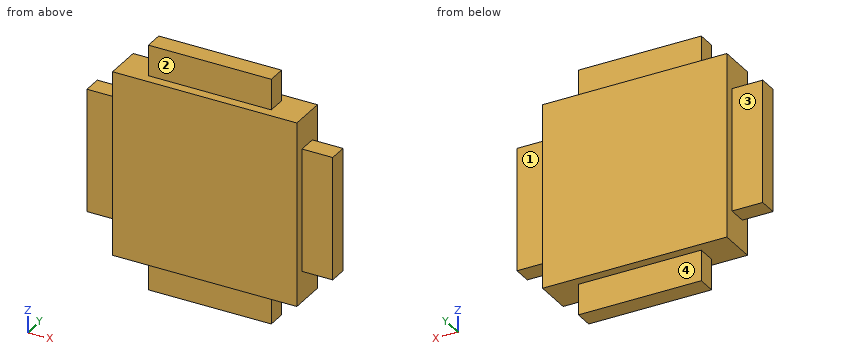
from build123d import *

# Parameters (mm, degrees)
SKETCH1_W                = 15
SKETCH1_H                = 15
BOSS_EXTRUDE2_DEPTH      = 3
SKETCH4_W                = 2.5
SKETCH4_H                = 10
SKETCH4_W_2              = 10
SKETCH4_H_2              = 2.5
BOSS_EXTRUDE3_DEPTH      = 0.75
BOSS_EXTRUDE3_DEPTH_BACK = 0.75


with BuildPart() as part:
    # Sketch1 → Boss-Extrude2 (new body)
    with BuildSketch(Plane(origin=(0, 0, 0), x_dir=(1, 0, 0), z_dir=(0, 1, 0))):
        Rectangle(SKETCH1_W, SKETCH1_H)
    extrude(amount=BOSS_EXTRUDE2_DEPTH)

    # Sketch4 → Boss-Extrude3 (add, two sides)
    with BuildSketch(Plane(origin=(0, 1.5, 0), x_dir=(1, 0, 0), z_dir=(0, 1, 0))) as boss_extrude3_sk:
        with Locations((-8.75, 0)):
            Rectangle(SKETCH4_W, SKETCH4_H)
        with Locations((0, -8.75)):
            Rectangle(SKETCH4_W_2, SKETCH4_H_2)
        with Locations((8.75, 0)):
            Rectangle(SKETCH4_W, SKETCH4_H)
        with Locations((0, 8.75)):
            Rectangle(SKETCH4_W_2, SKETCH4_H_2)
    extrude(amount=BOSS_EXTRUDE3_DEPTH)
    extrude(boss_extrude3_sk.sketch, amount=-BOSS_EXTRUDE3_DEPTH_BACK)


solid = part.part
Geometry: final body of the model. Coordinates: model frame, mm. Face numbers are marked on the shaded views. A direction names the side the tool comes from. Give positions to 0.01 mm unless a question says otherwise; leave off trailing zeros. Loops run counter-clockwise (first coordinate to the right, second up) from the corner with the lowest first, then second, coordinate; pieces in that order, holes last. Notation, with made-up numbers: (-16, 83.25) - (19, 83.25) arc R24 cw to (19, 122.25) - close; hole circle Ø10 at (-27, 36.5). An arc over 180 degrees is marked (long way). Answer as CSV lines item,"result". Start each with the question number.
1. Section B-B, the plane z = -1.75. Return loops of the section in (x, y), plus the area to 3 significant figures.
2. Pin query (flat end, axial travel): P1, Ø2, axis at x = -1.5, z = -9, coming from the -Y side; P2, Ø3, axis at x = -7, z = -1, coming from the -Y side; P3, Ø1.6, axis at y = 1.5, z = 8.5, coming from the -X side; P4, Ø1.2, axis at y = 1, z = -9.5, coming from the +X side. Return the tip coordinate at first contact, or that it passes through.
3. Ray query, L1, parallel to Z at x = -9, y = 2.15; L2, parallel to Z at x = -5, y = 2.3. Return the intervals inside material, ascending.
4. Section C-C, the plane y = 1.4. Return loops of the section in (x, z).
5. Reachability of the marked faces 1, 2, 3 and 4 from +Z, -Z, +X, -X, +Y, -Y: full face, straight path, thin tool, end or side. Return the list, or none.
6. Section A-A, the plane x = 2.25. Return loops of the section in (y, z), plus the area to 3 significant figures.
7. Section D-D, the plane z = 8.25. Return loops of the section in (x, y).
Answers:
1,outline,"(-10, 0.75) - (-7.5, 0.75) - (-7.5, 0) - (7.5, 0) - (7.5, 0.75) - (10, 0.75) - (10, 2.25) - (7.5, 2.25) - (7.5, 3) - (-7.5, 3) - (-7.5, 2.25) - (-10, 2.25) - close"
1,area,"52.5 mm2"
2,P1,"stops at y = 0.75"
2,P2,"stops at y = 0"
2,P3,"stops at x = -5"
2,P4,"stops at x = 5"
3,L1,"z = -5 to 5"
3,L2,"z = -7.5 to 7.5"
4,outline,"(-10, -5) - (-7.5, -5) - (-7.5, -7.5) - (-5, -7.5) - (-5, -10) - (5, -10) - (5, -7.5) - (7.5, -7.5) - (7.5, -5) - (10, -5) - (10, 5) - (7.5, 5) - (7.5, 7.5) - (5, 7.5) - (5, 10) - (-5, 10) - (-5, 7.5) - (-7.5, 7.5) - (-7.5, 5) - (-10, 5) - close"
5,face 1,"+Z, -Z, +X, +Y"
5,face 2,"+Z, +X, -X, -Y"
5,face 3,"+Z, -Z, -X, +Y"
5,face 4,"-Z, +X, -X, +Y"
6,outline,"(0, -7.5) - (0.75, -7.5) - (0.75, -10) - (2.25, -10) - (2.25, -7.5) - (3, -7.5) - (3, 7.5) - (2.25, 7.5) - (2.25, 10) - (0.75, 10) - (0.75, 7.5) - (0, 7.5) - close"
6,area,"52.5 mm2"
7,outline,"(-5, 0.75) - (5, 0.75) - (5, 2.25) - (-5, 2.25) - close"
